Build history of the part. All positions in model axes, mm. A direction names the side the tool comes from. Coordinates: 2 decimals unless noted, no trailing zeros. Write each loop counter-clockwise with the first axis right and the second up, starting at its lowest first coordinate (ties: lowest second). Pieces come first, ordered by that corner, then holes.
```python
from build123d import *

# Parameters (mm, degrees)
SKETCH1_W           = 54
SKETCH1_H           = 50
SKETCH1_R           = 2.6
BOSS_EXTRUDE1_DEPTH = 5
SKETCH2_W           = 4.8
SKETCH2_H           = 50
BOSS_EXTRUDE2_DEPTH = 44
SKETCH3_R           = 2.6
CUT_EXTRUDE1_DEPTH  = 10
FILLET1_R           = 25
CHAMFER1_SIZE       = 1
CHAMFER2_SIZE       = 1
CHAMFER3_SIZE       = 1


with BuildPart() as part:
    # Sketch1 → Boss-Extrude1 (new body)
    with BuildSketch(Plane.XY):
        with Locations((27, 25)):
            Rectangle(SKETCH1_W, SKETCH1_H)
        with Locations((5, 45)):
            Circle(SKETCH1_R, mode=Mode.SUBTRACT)
        with Locations((5, 5)):
            Circle(SKETCH1_R, mode=Mode.SUBTRACT)
    extrude(amount=BOSS_EXTRUDE1_DEPTH)

    # Sketch2 → Boss-Extrude2 (add)
    with BuildSketch(Plane.ZY.offset(-10)):
        with Locations((-2.4, 25)):
            Rectangle(SKETCH2_W, SKETCH2_H)
    extrude(amount=-BOSS_EXTRUDE2_DEPTH)

    # Sketch3 → Cut-Extrude1 (cut)
    with BuildSketch(Plane(origin=(0, 0, -4.8), x_dir=(-1, 0, 0), z_dir=(0, 0, -1))):
        with Locations(Location((-47.1, 25, 0), (0, 0, 90))):
            Circle(SKETCH3_R)
    extrude(amount=-CUT_EXTRUDE1_DEPTH, mode=Mode.SUBTRACT)

    # Fillet1
    fillet1_edges = [part.edges().sort_by_distance(p)[0] for p in [
        (54, 0, 0.1),
        (54, 50, 0.1),
    ]]
    fillet(fillet1_edges, radius=FILLET1_R - 0.0001)  # a hair under: the kernel refuses the full size

    # Chamfer1
    chamfer1_edges = [part.edges().sort_by_distance(p)[0] for p in [
        (47.1, 22.4, 5),
    ]]
    chamfer(chamfer1_edges, length=CHAMFER1_SIZE)

    # Chamfer2
    chamfer2_edges = [part.edges().sort_by_distance(p)[0] for p in [
        (14.50005, 50, 5),
        (46.677698819, 42.677698819, 5),
        (46.677698819, 7.322301181, 5),
        (14.50005, 0, 5),
    ]]
    chamfer(chamfer2_edges, length=CHAMFER2_SIZE)

    # Chamfer3
    chamfer3_edges = [part.edges().sort_by_distance(p)[0] for p in [
        (19.50005, 50, -4.8),
        (19.50005, 0, -4.8),
        (46.677698819, 42.677698819, -4.8),
        (46.677698819, 7.322301181, -4.8),
    ]]
    chamfer(chamfer3_edges, length=CHAMFER3_SIZE)


solid = part.part
```
1. Flat gauge pins, fed straight in: pin 1 (4 mm diameter, centred on x = 43.5, z = -2.5, fed in from -Y); pin 2 (3 mm diameter, centred on x = 7, y = 25.5, fed in from -Z); pin 3 (4 mm diameter, centred on x = 42.5, z = -2.5, fed in from +Y). Where does each tip first touch, or does it go through?
Computed values:
pin 1: stops at y = 3.35
pin 2: stops at z = 0
pin 3: stops at y = 47.2
2. Mould opens along Y. For faces 1 (the face through (46.27, 8.105, -4.64)), 2 (the face through (49.678, 24.662, -0.462)), 3 (the face through (45.895, 42.27, -4.64)), 4 (the face through (5, 25, 0)) say: +Y half, -Y half, draft (parallel to the pull), parting line (faces both ways), or undercut.
Computed values:
face 1: -Y half
face 2: undercut
face 3: +Y half
face 4: draft
3. Saw through at A-A on x = 5. List the corners of the cut face in (y, z), plus the area to 3 significant figures.
Computed values:
outline: (0, 0) - (2.4, 0) - (2.4, 5) - (1, 5) - (0, 4) - close; (7.6, 0) - (42.4, 0) - (42.4, 5) - (7.6, 5) - close; (47.6, 0) - (50, 0) - (50, 4) - (49, 5) - (47.6, 5) - close
area: 197 mm2
4. Saw through at B-B on z = 2. State how many separate pieces and enclosed holes the cut face has, plus the area to 3 significant figures.
Computed values:
separate pieces: 1
enclosed holes: 3
area: 2,370 mm2
5. 3-axis set-ups, long thin cutter, end or side, ignore diameter. For faces 5 (the face through (26, 25, 5)), 6 (the face through (10, 25, -2)): which of +Z, -Z, +X, -X, +Y, -Y reach the whole face in a straight line?
Computed values:
face 5: +Z, +X, -X, +Y, -Y
face 6: -Z, -X, +Y, -Y
6. Probe line 1 along Y through (x, z) = (5, 3.95); line 2 along X through (y, z) = (25, -1.25); line 3 along X through (y, z) = (25, 0.5). List the from-to ranges inside material, lowest first.
Computed values:
line 1: y = 0 to 2.4, 7.6 to 42.4, 47.6 to 50
line 2: x = 10 to 44.5, 49.7 to 54
line 3: x = 0 to 44.5, 49.7 to 54
